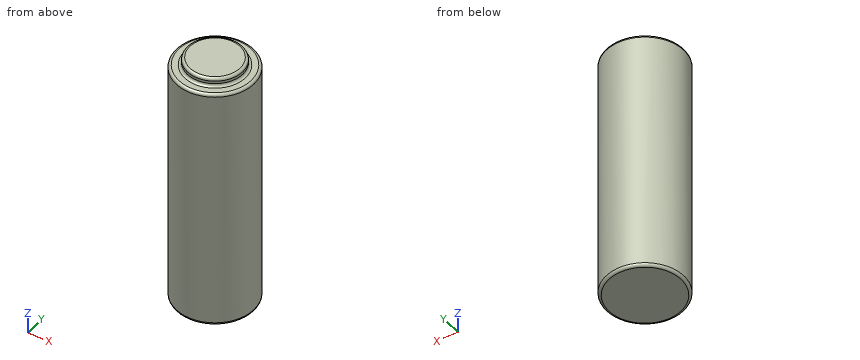
```python
from build123d import *

# Parameters (mm, degrees)
SKETCH1_R           = 7.400445615
BOSS_EXTRUDE1_DEPTH = 47.157501005
SKETCH2_R           = 5.279749884
BOSS_EXTRUDE2_DEPTH = 1.524
FILLET1_R           = 0.508
FILLET2_R           = 0.508
FILLET3_R           = 0.508


with BuildPart() as part:
    # Sketch1 → Boss-Extrude1 (new body)
    with BuildSketch(Plane.XY):
        with Locations((23.495, 8.89)):
            Circle(SKETCH1_R)
    extrude(amount=BOSS_EXTRUDE1_DEPTH)

    # Sketch2 → Boss-Extrude2 (add)
    with BuildSketch(Plane.XY.offset(47.157501005)):
        with Locations((23.495, 8.89)):
            Circle(SKETCH2_R)
    extrude(amount=BOSS_EXTRUDE2_DEPTH)

    # Fillet1
    fillet1_edges = [part.edges().sort_by_distance(p)[0] for p in [
        (18.215250116, 8.89, 48.681501005),
    ]]
    fillet(fillet1_edges, radius=FILLET1_R)

    # Fillet2
    fillet2_edges = [part.edges().sort_by_distance(p)[0] for p in [
        (16.094554385, 8.89, 47.157501005),
        (18.215250116, 8.89, 47.157501005),
    ]]
    fillet(fillet2_edges, radius=FILLET2_R)

    # Fillet3
    fillet3_edges = [part.edges().sort_by_distance(p)[0] for p in [
        (16.094554385, 8.89, 0),
    ]]
    fillet(fillet3_edges, radius=FILLET3_R)


solid = part.part
```
Design review of the part built by this model. Coordinates are the model's own, in mm. Coordinates: 2 decimals unless noted, no trailing zeros. Order: outer loops, then holes, each group sorted by start corner. A loop starts at its lowest first (then second) coordinate and runs counter-clockwise, first axis right, second up. Notation, with made-up numbers: M -23,-9 L -19,-9 A26 ccw -19,27 Z; hole C 20,63 d1. An arc over 180 degrees is marked long. Answer as a JSON object with one key per item and string values. Group by question number.
1) Wall thickness on L1, parallel to Z at x = 25.5, y = 14.5; L2, parallel to Y at x = 20.25, z = 19.5; L3, parallel to Y at x = 27, z = 34: over which ranges is each line inside the solid? List them lowest first.
2) Add section A-A, the plane z = 25.5. Write out the cut boundary in (x, y) (3 decimals).
3) For pin 1 (4 mm diameter, centred on x = 27, z = 21, fed in from -Y); pin 2 (1.5 mm diameter, centred on y = 11.5, z = 40.5, fed in from -X); pin 3 (5 mm diameter, centred on x = 19, z = 30.5, fed in from +Y), all flat-tipped, find the tip position at first contact; note any pin that passes through.
Computed values:
{
 "1": {"L1": "z = 0 to 47.16", "L2": "y = 2.24 to 15.54", "L3": "y = 2.37 to 15.41"},
 "2": {"outline": "C 23.495,8.89 d14.801"},
 "3": {"pin 1": "stops at y = 1.64", "pin 2": "stops at x = 16.33", "pin 3": "stops at y = 16.02"}
}
